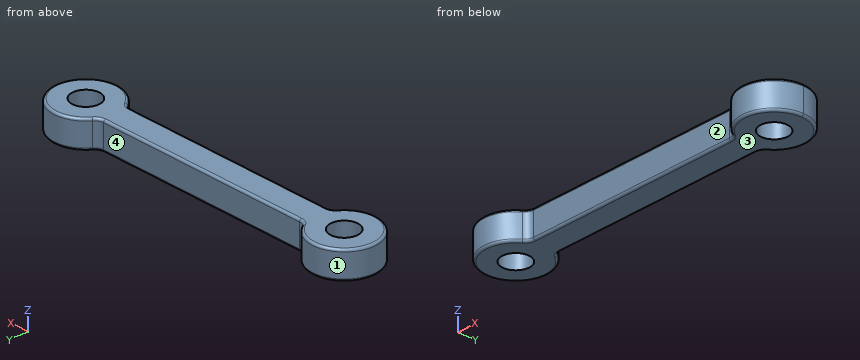
```python
from build123d import *

# Parameters (mm, degrees)
SKETCH3_R           = 1.5
BOSS_EXTRUDE2_DEPTH = 3
FILLET1_R           = 1
FILLET2_R           = 0.25


with BuildPart() as part:
    # Sketch3 → Boss-Extrude2 (new body)
    # profile 1 of 5: a face of its own
    with BuildSketch(Plane.XY):
        with BuildLine():
            ThreePointArc((3.16227766, 1.5), (-3.5, 0), (3.16227766, -1.5))
            Line((3.16227766, -1.5), (3.16227766, 1.5))
        make_face()
        Circle(SKETCH3_R, mode=Mode.SUBTRACT)
    # profile 2 of 5: a face of its own
    with BuildSketch(Plane.XY):
        with BuildLine():
            Line((3.16227766, 1.5), (3.16227766, -1.5))
            ThreePointArc((3.16227766, -1.5), (3.414525722, -0.768774411), (3.5, 0))
            ThreePointArc((3.5, 0), (3.414525722, 0.768774411), (3.16227766, 1.5))
        make_face()
    # profile 3 of 5: a face of its own
    with BuildSketch(Plane.XY):
        with BuildLine():
            Line((3.16227766, -1.5), (27.83772234, -1.5))
            ThreePointArc((27.83772234, -1.5), (27.5, 0), (27.83772234, 1.5))
            Line((27.83772234, 1.5), (3.16227766, 1.5))
            ThreePointArc((3.16227766, 1.5), (3.414525722, 0.768774411), (3.5, 0))
            ThreePointArc((3.5, 0), (3.414525722, -0.768774411), (3.16227766, -1.5))
        make_face()
    # profile 4 of 5: a face of its own
    with BuildSketch(Plane.XY):
        with BuildLine():
            Line((27.83772234, 1.5), (27.83772234, -1.5))
            ThreePointArc((27.83772234, -1.5), (31.768774411, -3.414525722), (34.5, 0))
            ThreePointArc((34.5, 0), (31.768774411, 3.414525722), (27.83772234, 1.5))
        make_face()
        with Locations((31, 0)):
            Circle(SKETCH3_R, mode=Mode.SUBTRACT)
    # profile 5 of 5: a face of its own
    with BuildSketch(Plane.XY):
        with BuildLine():
            ThreePointArc((27.83772234, 1.5), (27.5, 0), (27.83772234, -1.5))
            Line((27.83772234, -1.5), (27.83772234, 1.5))
        make_face()
    extrude(amount=BOSS_EXTRUDE2_DEPTH)

    # Fillet1
    fillet1_edges = [part.edges().sort_by_distance(p)[0] for p in [
        (3.16227766, 1.5, 1.5),
        (27.83772234, 1.5, 1.5),
        (27.83772234, -1.5, 1.5),
        (3.16227766, -1.5, 1.5),
    ]]
    fillet(fillet1_edges, radius=FILLET1_R)

    # Fillet2
    fillet2_edges = [part.edges().sort_by_distance(p)[0] for p in [
        (15.5, -1.5, 0),
        (15.5, -1.5, 3),
        (-3.5, 0, 0),
        (-3.5, 0, 3),
        (15.5, 1.5, 0),
        (15.5, 1.5, 3),
        (34.5, 0, 0),
        (34.5, 0, 3),
        (3.270252866, -1.618082896, 0),
        (3.270252866, -1.618082896, 3),
        (3.270252866, 1.618082896, 0),
        (3.270252866, 1.618082896, 3),
        (27.729747134, 1.618082896, 0),
        (27.729747134, 1.618082896, 3),
        (27.729747134, -1.618082896, 0),
        (27.729747134, -1.618082896, 3),
    ]]
    fillet(fillet2_edges, radius=FILLET2_R)


solid = part.part
```
The listing builds one solid part. Answer for the finished solid, in the listing's coordinates (mm). Face numbers are marked on the shaded views. A direction names the side the tool comes from. Coordinates: 2 decimals unless noted, no trailing zeros. Loops run counter-clockwise (first coordinate to the right, second up) from the corner with the lowest first, then second, coordinate; pieces in that order, holes last. Notation, with made-up numbers: (-31, 23.25) -> (6, 23.25) arc R18 ccw to (6, 41.25) -> close; hole circle Ø1 at (-32.5, 87). An arc over 180 degrees is marked (long way). Use one line per item in the form item = value. Start each with the question number.
Item 1: The part is cut by section A-A on z = 0.65. Determine the outline of the cut face in (x, y), then the cut area to 3 significant figures.
Item 2: The part is cut by section B-B on x = 14. Determine the outline of the cut face in (y, z).
Item 3: The mould has two halves that part along X. Classify the marked faces 3 and 4: released by +X, released by -X, zero draft, split by the parting line, or undercut.
Item 4: Flat-ended cylindrical pins translate along their axes: pin 1 Ø1 at (x, z) = (7.5, 2.5) entering from -Y; pin 2 Ø1.5 at (x, y) = (25, 1.5) entering from -Z; pin 3 Ø0.8 at (x, z) = (15.5, 2) entering from +Y. Find the tip coordinate at first contact, or state that the pin passes through.
Item 5: Consider L1, parallel to Y at x = 0, z = 2.4; L2, parallel to X at y = -0.25, z = 0.85; L3, parallel to X at y = -1.25, z = 1.7. Determine where each line is inside the solid, lowest interval first. Write a range as [from, to].
Item 6: A tool of negligible diameter and unlimited length cuts with its end or side. For the marked faces 1 and 2, from which of +Z, -Z, +X, -X, +Y, -Y can it reach the whole face along a straight path? Write none if from no direction.
Item 7: The part is cut by section C-C on y = -0.75. Count the separate pieces of the cut face and the enclosed holes in it, then the cut area to 3 significant figures.
Answer key:
q1.outline = (2.91, -1.94) arc R1 cw to (3.74, -1.5) -> (27.26, -1.5) arc R1 cw to (28.09, -1.94) arc R3.5 ccw (long way) to (28.09, 1.94) arc R1 cw to (27.26, 1.5) -> (3.74, 1.5) arc R1 cw to (2.91, 1.94) arc R3.5 ccw (long way) to start; hole circle Ø3 at (0, 0); hole circle Ø3 at (31, 0)
q1.area = 136 mm2
q2.outline = (-1.5, 0.25) arc R0.25 ccw to (-1.25, 0) -> (1.25, 0) arc R0.25 ccw to (1.5, 0.25) -> (1.5, 2.75) arc R0.25 ccw to (1.25, 3) -> (-1.25, 3) arc R0.25 ccw to (-1.5, 2.75) -> close
q3.face_3 = zero draft
q3.face_4 = undercut
q4.pin_1 = -1.5
q4.pin_2 = 0
q4.pin_3 = 1.5
q5.L1 = [-3.5, -1.5], [1.5, 3.5]
q5.L2 = [-3.49, -1.48], [1.48, 29.52], [32.48, 34.49]
q5.L3 = [-3.27, -0.83], [0.83, 30.17], [31.83, 34.27]
q6.face_1 = +Z, -Z
q6.face_2 = +Z, -Z, -Y
q7.separate_pieces = 3
q7.enclosed_holes = 0
q7.area = 97.9 mm2
